from build123d import *

# Parameters (mm, degrees)
SKETCH1_R      = 3.4
EXTRUDE1_DEPTH = 300


with BuildPart() as part:
    # Sketch1 → Extrude1 (new body)
    with BuildSketch(Plane.XY):
        with BuildLine():
            Line((3.414141554, 7.7), (-3.414141554, 7.7))
            ThreePointArc((-3.414141554, 7.7), (-5.219014233, 8.062418522), (-6.750527179, 9.083878589))
            Line((-6.750527179, 9.083878589), (-10.040658191, 12.367344817))
            ThreePointArc((-10.040658191, 12.367344817), (-10.221657959, 12.649942114), (-10.285, 12.979502327))
            Line((-10.285, 12.979502327), (-10.285, 15.292928509))
            ThreePointArc((-10.285, 15.292928509), (-9.913025612, 16.190954121), (-9.015, 16.562928509))
            Line((-9.015, 16.562928509), (-6.771827505, 16.562928509))
            Line((-6.771827505, 16.562928509), (-6.771827505, 15.94))
            Line((-6.771827505, 15.94), (-5.6348, 15.94))
            ThreePointArc((-5.6348, 15.94), (-4.521248241, 16.401248241), (-4.06, 17.5148))
            Line((-4.06, 17.5148), (-4.06, 18.4252))
            ThreePointArc((-4.06, 18.4252), (-4.521248241, 19.538751759), (-5.6348, 20))
            Line((-5.6348, 20), (-13.0175, 20))
            Line((-13.0175, 20), (-16.825, 20))
            ThreePointArc((-16.825, 20), (-19.07006403, 19.07006403), (-20, 16.825))
            Line((-20, 16.825), (-20, -16.825))
            ThreePointArc((-20, -16.825), (-19.07006403, -19.07006403), (-16.825, -20))
            Line((-16.825, -20), (-13.0175, -20))
            Line((-13.0175, -20), (-5.6348, -20))
            ThreePointArc((-5.6348, -20), (-4.521248241, -19.538751759), (-4.06, -18.4252))
            Line((-4.06, -18.4252), (-4.06, -17.5148))
            ThreePointArc((-4.06, -17.5148), (-4.521248241, -16.401248241), (-5.6348, -15.94))
            Line((-5.6348, -15.94), (-6.893826419, -15.94))
            Line((-6.893826419, -15.94), (-6.893826419, -16.702464473))
            Line((-6.893826419, -16.702464473), (-9.015, -16.702464473))
            ThreePointArc((-9.015, -16.702464473), (-9.913025612, -16.330490085), (-10.285, -15.432464473))
            Line((-10.285, -15.432464473), (-10.285, -12.948084155))
            ThreePointArc((-10.285, -12.948084155), (-10.217156337, -12.607462266), (-10.023980268, -12.318829212))
            Line((-10.023980268, -12.318829212), (-6.773258234, -9.074692133))
            ThreePointArc((-6.773258234, -9.074692133), (-5.238079583, -8.057096539), (-3.431215906, -7.7))
            Line((-3.431215906, -7.7), (3.431215906, -7.7))
            ThreePointArc((3.431215906, -7.7), (5.238079583, -8.057096539), (6.773258234, -9.074692133))
            Line((6.773258234, -9.074692133), (10.023980268, -12.318829212))
            ThreePointArc((10.023980268, -12.318829212), (10.217156337, -12.607462266), (10.285, -12.948084155))
            Line((10.285, -12.948084155), (10.285, -15.432464473))
            ThreePointArc((10.285, -15.432464473), (9.913025612, -16.330490085), (9.015, -16.702464473))
            Line((9.015, -16.702464473), (6.893826419, -16.702464473))
            Line((6.893826419, -16.702464473), (6.893826419, -15.94))
            Line((6.893826419, -15.94), (5.6348, -15.94))
            ThreePointArc((5.6348, -15.94), (4.521248241, -16.401248241), (4.06, -17.5148))
            Line((4.06, -17.5148), (4.06, -18.4252))
            ThreePointArc((4.06, -18.4252), (4.521248241, -19.538751759), (5.6348, -20))
            Line((5.6348, -20), (13.0175, -20))
            Line((13.0175, -20), (16.825, -20))
            ThreePointArc((16.825, -20), (19.07006403, -19.07006403), (20, -16.825))
            Line((20, -16.825), (20, 16.825))
            ThreePointArc((20, 16.825), (19.07006403, 19.07006403), (16.825, 20))
            Line((16.825, 20), (13.0175, 20))
            Line((13.0175, 20), (5.6348, 20))
            ThreePointArc((5.6348, 20), (4.521248241, 19.538751759), (4.06, 18.4252))
            Line((4.06, 18.4252), (4.06, 17.5148))
            ThreePointArc((4.06, 17.5148), (4.521248241, 16.401248241), (5.6348, 15.94))
            Line((5.6348, 15.94), (6.771827505, 15.94))
            Line((6.771827505, 15.94), (6.771827505, 16.562928509))
            Line((6.771827505, 16.562928509), (9.015, 16.562928509))
            ThreePointArc((9.015, 16.562928509), (9.913025612, 16.190954121), (10.285, 15.292928509))
            Line((10.285, 15.292928509), (10.285, 12.979502327))
            ThreePointArc((10.285, 12.979502327), (10.221657959, 12.649942114), (10.040658191, 12.367344817))
            Line((10.040658191, 12.367344817), (6.750527179, 9.083878589))
            ThreePointArc((6.750527179, 9.083878589), (5.219014233, 8.062418522), (3.414141554, 7.7))
        make_face()
        Circle(SKETCH1_R, mode=Mode.SUBTRACT)
        with BuildLine():
            Line((-12.564539323, -18.35), (-15.5575, -18.35))
            ThreePointArc((-15.5575, -18.35), (-17.531656749, -17.531656749), (-18.35, -15.5575))
            Line((-18.35, -15.5575), (-18.35, 15.5575))
            ThreePointArc((-18.35, 15.5575), (-17.531656749, 17.531656749), (-15.5575, 18.35))
            Line((-15.5575, 18.35), (-12.566039323, 18.35))
            ThreePointArc((-12.566039323, 18.35), (-12.121960893, 18.165032537), (-11.935, 17.721789669))
            Line((-11.935, 17.721789669), (-11.935, 10.955500711))
            ThreePointArc((-11.935, 10.955500711), (-11.692410278, 9.694593073), (-10.97025746, 8.632880704))
            Line((-10.97025746, 8.632880704), (-9.032953263, 6.699500885))
            ThreePointArc((-9.032953263, 6.699500885), (-8.018239143, 5.133591891), (-7.685, 3.297654148))
            Line((-7.685, 3.297654148), (-7.685, -3.50798046))
            ThreePointArc((-7.685, -3.50798046), (-8.092979352, -5.282450357), (-9.138589048, -6.773051218))
            Line((-9.138589048, -6.773051218), (-11.073928072, -8.704469846))
            ThreePointArc((-11.073928072, -8.704469846), (-11.72635669, -9.745106152), (-11.935, -10.955500711))
            Line((-11.935, -10.955500711), (-11.935, -17.721789669))
            ThreePointArc((-11.935, -17.721789669), (-12.121425838, -18.164510172), (-12.564539323, -18.35))
        make_face(mode=Mode.SUBTRACT)
        with BuildLine():
            Line((11.935, -10.955500711), (11.935, -17.721789669))
            ThreePointArc((11.935, -17.721789669), (12.121425838, -18.164510172), (12.564539323, -18.35))
            Line((12.564539323, -18.35), (15.5575, -18.35))
            ThreePointArc((15.5575, -18.35), (17.531656749, -17.531656749), (18.35, -15.5575))
            Line((18.35, -15.5575), (18.35, 15.5575))
            ThreePointArc((18.35, 15.5575), (17.531656749, 17.531656749), (15.5575, 18.35))
            Line((15.5575, 18.35), (12.566039323, 18.35))
            ThreePointArc((12.566039323, 18.35), (12.121960893, 18.165032537), (11.935, 17.721789669))
            Line((11.935, 17.721789669), (11.935, 10.955500711))
            ThreePointArc((11.935, 10.955500711), (11.692410278, 9.694593073), (10.97025746, 8.632880704))
            Line((10.97025746, 8.632880704), (9.032953263, 6.699500885))
            ThreePointArc((9.032953263, 6.699500885), (8.018239143, 5.133591891), (7.685, 3.297654148))
            Line((7.685, 3.297654148), (7.685, -3.50798046))
            ThreePointArc((7.685, -3.50798046), (8.092979352, -5.282450357), (9.138589048, -6.773051218))
            Line((9.138589048, -6.773051218), (11.073928072, -8.704469846))
            ThreePointArc((11.073928072, -8.704469846), (11.72635669, -9.745106152), (11.935, -10.955500711))
        make_face(mode=Mode.SUBTRACT)
    extrude(amount=-EXTRUDE1_DEPTH)


solid = part.part
Work out the finished part from the listing and answer in its coordinate system (mm). A direction names the side the tool comes from. Coordinates: 2 decimals unless noted, no trailing zeros. Write each loop counter-clockwise with the first axis right and the second up, starting at its lowest first coordinate (ties: lowest second). Pieces come first, ordered by that corner, then holes. Notation, with made-up numbers: M 5.25,70.25 L 42.25,70.25 A15 ccw 42.25,79.25 Z; hole C -22,15 d8. An arc over 180 degrees is marked long. Use one line per item in the form item = value. Start each with the question number.
1. The part is cut by section C-C (z = -162.5). Give the number of separate pieces and of enclosed holes in the cut face, plus the area to 3 significant figures.
2. The part is cut by section B-B (x = 0). Give the vertices of the cut face in (y, z).
3. The mould has two halves that part along Y. Classify faces 4 (the face through (11, -20, -148)), 5 (the face through (-2, 3, -300)), 6 (the face through (-11.935, -14, -148)): released by +Y, released by -Y, zero draft, split by the parting line, or undercut.
4. A tool of negligible diameter and unlimited length cuts with its end or side. For faces 1 (the face through (-7.685, 0, -148)), 2 (the face through (0, -7.7, -148)), 3 (the face through (0, 7.7, -148)), from which of +Z, -Z, +X, -X, +Y, -Y can it reach the whole face along a straight path? Write none if from no direction.
5. The part is cut by section A-A (y = 0). Give the vertices of the cut face in (x, z) (3 decimals), plus the area to 3 significant figures.
6. Straight lines are drawn through the part: probe 1 along X at (y, z) = (15, -277.5) (3 decimals); probe 2 along X at (y, z) = (10, -244); probe 3 along Y at (x, z) = (0, -139). For each, find the intervals that lie inside material, in ascending order. Write a range as from..to.
7. Each of these flat-tipped pins is pushed along its axis until it touches: P1, Ø1, axis at y = 18, z = -169.5, coming from the -X side; P2, Ø7.5, axis at x = -1, z = -189, coming from the +Y side; P3, Ø2, axis at x = 1.5, z = -127.5, coming from the -Y side. Where does it stop, or does it pass through?
Evaluation:
q1.separate_pieces = 1
q1.enclosed_holes = 3
q1.area = 598 mm^2
q2.outline = M -7.7,-300 L -3.4,-300 L -3.4,0 L -7.7,0 Z; M 3.4,-300 L 7.7,-300 L 7.7,0 L 3.4,0 Z
q3.face_4 = released by -Y
q3.face_5 = zero draft
q3.face_6 = undercut
q4.face_1 = +Z, -Z
q4.face_2 = +Z, -Z, -Y
q4.face_3 = +Z, -Z, +Y
q5.outline = M -20,-300 L -18.35,-300 L -18.35,0 L -20,0 Z; M -7.685,-300 L -3.4,-300 L -3.4,0 L -7.685,0 Z; M 3.4,-300 L 7.685,-300 L 7.685,0 L 3.4,0 Z; M 18.35,-300 L 20,-300 L 20,0 L 18.35,0 Z
q5.area = 3,560 mm^2
q6.probe_1 = -20..-18.35, -11.935..-10.285, 10.285..11.935, 18.35..20
q6.probe_2 = -20..-18.35, -11.8..-7.67, 7.67..11.8, 18.35..20
q6.probe_3 = -7.7..-3.4, 3.4..7.7
q7.P1 = -19.93
q7.P2 = 19.73
q7.P3 = -7.7
